Build history of the part. All positions in model axes, mm. A direction names the side the tool comes from. Coordinates: 2 decimals unless noted, no trailing zeros. Loops run counter-clockwise (first coordinate to the right, second up) from the corner with the lowest first, then second, coordinate; pieces in that order, holes last.
(1) Wall check: L1, parallel to Z at x = 6, y = -9.5; L2, parallel to Y at x = -4.5, z = 3.25; L3, parallel to Y at x = -4, z = 12. Give the ranges that are in metal, low to high.
(2) Two-plate mould, pull along X, no slides. Class faces 3 (the face through (1.08, -4.88, 10.54)), 4 (the face through (0.4, -13.3, 0)), 5 (the face through (4.9, -22.08, 14.16)): pulls with the +X half, pulls with the -X half, needs draft (parallel to the pull), parting line crosses it, or undercut.
(3) Tool access for faces 1 (the face through (-5, -5, 15)), 2 (the face through (-5, -2, 7.5)): list every direction of +Z, -Z, +X, -X, +Y, -Y with a clear straight run to the whole face (end or side of a thin tool).
(4) Slice it at A-A (y = 0). Give the cut face in (x, z), and give its area (3 significant figures).
(5) Slice it at C-C (z = 3.5). Give the cut face in (x, y), and give its area (3 significant figures).
(6) Flat gauge pins, fed straight in: P1, Ø3, axis at x = -2, z = 13, coming from the +Y side; P2, Ø6, axis at x = -1, z = 8, coming from the -Y side; P3, Ø3, axis at x = -24.5, z = 8.5, coming from the +Y side; P4, Ø8, axis at x = 13.5, y = -21, coming from the +Z side. Where does each tip first touch, or does it go through?
from build123d import *

# Parameters (mm, degrees)
F2_SIZE = 2
F3_SIZE = 1.5
F4_SIZE = 1.5


with BuildPart() as f1:
    # F0 (on Front) → F1 (revolve)
    with BuildSketch(Plane.XZ):
        Polygon((-33, 0), (-11.5, 0), (-11.5, 7.5), (-5, 7.5), (-5, 15), (-22, 15), align=None)
    revolve(axis=Axis((0, 0, 3.75), (0, 0, -1)))

    # F2
    f2_edges = [f1.edges().sort_by_distance(p)[0] for p in [
        (33, 0, 0),
    ]]
    chamfer(f2_edges, length=F2_SIZE)

    # F3
    f3_edges = [f1.edges().sort_by_distance(p)[0] for p in [
        (5, 0, 15),
    ]]
    chamfer(f3_edges, length=F3_SIZE)

    # F4
    f4_edges = [f1.edges().sort_by_distance(p)[0] for p in [
        (11.5, 0, 0),
    ]]
    chamfer(f4_edges, length=F4_SIZE)


solid = f1.part
Response values:
1. L1: z = 7.5 to 15
1. L2: y = -30.28 to -10.58, 10.58 to 30.28
1. L3: y = -23.87 to -3, 3 to 23.87
2. face 3: undercut
2. face 4: needs draft
2. face 5: parting line crosses it
3. face 1: +Z, +X, -X, +Y, -Y
3. face 2: -Z
4. outline: (-31.82, 1.61) - (-31, 0) - (-13, 0) - (-11.5, 1.5) - (-11.5, 7.5) - (-5, 7.5) - (-5, 13.5) - (-6.5, 15) - (-22, 15) - close; (5, 7.5) - (11.5, 7.5) - (11.5, 1.5) - (13, 0) - (31, 0) - (31.82, 1.61) - (22, 15) - (6.5, 15) - (5, 13.5) - close
4. area: 570 mm2
5. outline: circle Ø60.87 at (0, 0); hole circle Ø23 at (0, 0)
5. area: 2,490 mm2
6. P1: stops at y = 24.49
6. P2: stops at y = -29.32
6. P3: stops at y = 14.48
6. P4: stops at z = 15
